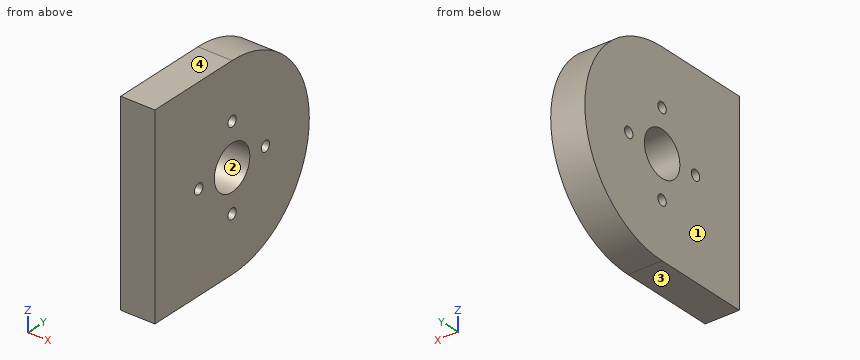
from build123d import *

# Parameters (mm, degrees)
SKETCH1_W               = 50
SKETCH1_H               = 150
BOSS_EXTRUDE1_DEPTH     = 55
CUT_EXTRUDE1_DEPTH      = 168.406690428
CUT_EXTRUDE1_DEPTH_BACK = 45
SKETCH2_R               = 10.25
SKETCH7_R               = 1
SKETCH7_R_2             = 4.25
CUT_EXTRUDE3_DEPTH      = 10
SKETCH8_W               = 55
SKETCH8_H               = 55
SKETCH8_R               = 10.25
BOSS_EXTRUDE2_DEPTH     = 50
SKETCH10_W              = 8
SKETCH10_H              = 10.25
SKETCH10_W_2            = 17
SKETCH10_H_2            = 1
SKETCH10_W_3            = 34
SKETCH10_H_3            = 20
SKETCH10_H_4            = 5
CUT_EXTRUDE4_DEPTH      = 214.717102732
SKETCH11_W              = 34
SKETCH11_H              = 13.25
BOSS_EXTRUDE4_DEPTH     = 25
SKETCH13_W              = 55
SKETCH13_H              = 10
CUT_EXTRUDE5_DEPTH      = 8
SKETCH14_R              = 5.030159043
CUT_EXTRUDE6_DEPTH      = 8
SKETCH15_W              = 34
SKETCH15_H              = 0.25
BOSS_EXTRUDE5_DEPTH     = 13.25
CUT_EXTRUDE7_DEPTH      = 181.416185527
BOSS_EXTRUDE6_START     = 1.5
SKETCH19_R              = 10.25
SKETCH19_R_2            = 1
SKETCH19_R_3            = 4.25
BOSS_EXTRUDE6_DEPTH     = 1.5
CUT_EXTRUDE8_DEPTH      = 184.89467094
SKETCH21_R              = 5.030159043
SKETCH21_R_2            = 4.5
BOSS_EXTRUDE7_DEPTH     = 8
SKETCH24_W              = 4
SKETCH24_H              = 30
CUT_EXTRUDE10_DEPTH     = 181.416185527
SKETCH25_W              = 55
SKETCH25_H              = 86.25
CUT_EXTRUDE11_DEPTH     = 4
BOSS_EXTRUDE8_START     = 4
SKETCH26_R              = 1
SKETCH26_R_2            = 4.25
BOSS_EXTRUDE8_DEPTH     = 4
SKETCH27_W              = 4
SKETCH27_H              = 123.25
CUT_EXTRUDE12_DEPTH     = 181.416185527
CUT_EXTRUDE13_DEPTH     = 180.905530765
SKETCH29_W              = 42
SKETCH29_H              = 9
CUT_EXTRUDE15_DEPTH     = 174.776436838
SKETCH30_R              = 4.5
SKETCH30_R_2            = 1.45
BOSS_EXTRUDE9_DEPTH     = 4
SKETCH31_W              = 37
SKETCH31_H              = 55
CUT_EXTRUDE16_DEPTH     = 182.05247858
SKETCH32_W              = 73.968301754
SKETCH32_H              = 92.223299302
CUT_EXTRUDE17_DEPTH     = 182.05247858


with BuildPart() as part:
    # Sketch1 → Boss-Extrude1 (new body)
    with BuildSketch(Plane.XY):
        with Locations((0, -75)):
            Rectangle(SKETCH1_W, SKETCH1_H)
    extrude(amount=-BOSS_EXTRUDE1_DEPTH)

    # Sketch2 → Cut-Extrude1 (cut, two sides: drawn at the far end of the back side and taken through both)
    with BuildSketch(Plane(origin=(25, 0, 0), x_dir=(0, 0, -1), z_dir=(1, 0, 0)).offset(-CUT_EXTRUDE1_DEPTH_BACK)):
        with Locations(Location((27.5, -25, 0), (0, 0, 270))):
            Circle(SKETCH2_R)
    extrude(amount=CUT_EXTRUDE1_DEPTH + CUT_EXTRUDE1_DEPTH_BACK, mode=Mode.SUBTRACT)

    # Sketch7 → Cut-Extrude3 (cut)
    with BuildSketch(Plane(origin=(-20, 0, 0), x_dir=(0, 0, -1), z_dir=(1, 0, 0))):
        with Locations(Location((27.5, -17, 0), (0, 0, 90))):
            Circle(SKETCH7_R)
        with Locations(Location((35.5, -25, 0), (0, 0, 90))):
            Circle(SKETCH7_R)
        with Locations(Location((27.5, -33, 0), (0, 0, 90))):
            Circle(SKETCH7_R)
        with Locations(Location((19.5, -25, 0), (0, 0, 90))):
            Circle(SKETCH7_R)
        with Locations(Location((27.5, -25, 0), (0, 0, 90))):
            Circle(SKETCH7_R_2)
    extrude(amount=-CUT_EXTRUDE3_DEPTH, mode=Mode.SUBTRACT)

    # Sketch8 → Boss-Extrude2 (add)
    with BuildSketch(Plane(origin=(25, 0, 0), x_dir=(0, 0, -1), z_dir=(1, 0, 0))):
        with Locations((27.5, -177.5)):
            Rectangle(SKETCH8_W, SKETCH8_H)
        with Locations(Location((27.5, -180, 0), (0, 0, 90))):
            Circle(SKETCH8_R, mode=Mode.SUBTRACT)
    extrude(amount=-BOSS_EXTRUDE2_DEPTH)

    # Sketch10 → Cut-Extrude4 (cut, through all)
    with BuildSketch(Plane.XY):
        Polygon((-17, -205), (17, -205), (17, -191.25), (0, -191.25), (-17, -191.25), align=None)
        Polygon((-25, -205), (-17, -205), (-17, -191.25), (-17, -190.25), (-25, -190.25), align=None)
        Polygon((17, -191.25), (17, -205), (25, -205), (25, -190.25), (17, -190.25), align=None)
        with Locations((-21, -185.125)):
            Rectangle(SKETCH10_W, SKETCH10_H)
        with Locations((-21, -174.875)):
            Rectangle(SKETCH10_W, SKETCH10_H)
        with Locations((21, -174.875)):
            Rectangle(SKETCH10_W, SKETCH10_H)
        with Locations((21, -185.125)):
            Rectangle(SKETCH10_W, SKETCH10_H)
        with Locations((-8.5, -185.125)):
            Rectangle(SKETCH10_W_2, SKETCH10_H)
        with Locations((8.5, -185.125)):
            Rectangle(SKETCH10_W_2, SKETCH10_H)
        Polygon((0, -180), (17, -180), (17, -169.75), (-17, -169.75), (-17, -180), align=None)
        with Locations((-8.5, -190.75)):
            Rectangle(SKETCH10_W_2, SKETCH10_H_2)
        with Locations((8.5, -190.75)):
            Rectangle(SKETCH10_W_2, SKETCH10_H_2)
        with Locations((0, -154.75)):
            Rectangle(SKETCH10_W_3, SKETCH10_H_3)
        with Locations((0, -167.25)):
            Rectangle(SKETCH10_W_3, SKETCH10_H_4)
    extrude(amount=-CUT_EXTRUDE4_DEPTH, mode=Mode.SUBTRACT)

    # Sketch11 → Boss-Extrude4 (add)
    with BuildSketch(Plane.XZ.offset(144.75)):
        with Locations((0, -6.625)):
            Rectangle(SKETCH11_W, SKETCH11_H)
        with Locations((0, -48.375)):
            Rectangle(SKETCH11_W, SKETCH11_H)
    extrude(amount=BOSS_EXTRUDE4_DEPTH)

    # Sketch13 → Cut-Extrude5 (cut)
    with BuildSketch(Plane(origin=(25, 0, 0), x_dir=(0, 0, -1), z_dir=(1, 0, 0))):
        with Locations((27.5, -164.75)):
            Rectangle(SKETCH13_W, SKETCH13_H)
    cut_extrude5 = extrude(amount=-CUT_EXTRUDE5_DEPTH, mode=Mode.SUBTRACT)

    # Mirror2: Cut-Extrude5 across plane
    add(cut_extrude5.mirror(Plane(origin=(0, 0, 0), x_dir=(0, 0, 1), z_dir=(1, 0, 0))), mode=Mode.SUBTRACT)

    # Sketch14 → Cut-Extrude6 (cut)
    with BuildSketch(Plane(origin=(25, 0, 0), x_dir=(0, 0, -1), z_dir=(1, 0, 0))):
        with Locations(Location((16.5, -148, 0), (0, 0, 90))):
            Circle(SKETCH14_R)
        with Locations(Location((38.5, -148, 0), (0, 0, 90))):
            Circle(SKETCH14_R)
    cut_extrude6 = extrude(amount=-CUT_EXTRUDE6_DEPTH, mode=Mode.SUBTRACT)

    # Mirror3: Cut-Extrude6 across plane
    add(cut_extrude6.mirror(Plane(origin=(0, 0, 0), x_dir=(0, 0, 1), z_dir=(1, 0, 0))), mode=Mode.SUBTRACT)

    # Sketch15 → Boss-Extrude5 (add)
    with BuildSketch(Plane.XY):
        with Locations((0, -169.875)):
            Rectangle(SKETCH15_W, SKETCH15_H)
    boss_extrude5 = extrude(amount=-BOSS_EXTRUDE5_DEPTH)

    # Mirror4: Boss-Extrude5 across plane
    add(boss_extrude5.mirror(Plane.XY.offset(-27.5)))

    # Sketch16 → Cut-Extrude7 (cut, through all)
    with BuildSketch(Plane.XY):
        Polygon((-18.5, 0), (-18.5, -14.75), (-18.5, -35.25), (-18.5, -43.5), (25, -43.5), (25, 0), align=None)
    extrude(amount=-CUT_EXTRUDE7_DEPTH, mode=Mode.SUBTRACT)

    # Sketch19 → Boss-Extrude6 (add)
    with BuildSketch(Plane(origin=(-20, 0, 0), x_dir=(0, 0, -1), z_dir=(1, 0, 0)).offset(BOSS_EXTRUDE6_START)):
        with Locations((27.5, -25)):
            Circle(SKETCH19_R)
        with Locations(Location((27.5, -17, 0), (0, 0, 90))):
            Circle(SKETCH19_R_2, mode=Mode.SUBTRACT)
        with Locations(Location((27.5, -33, 0), (0, 0, 90))):
            Circle(SKETCH19_R_2, mode=Mode.SUBTRACT)
        with Locations(Location((19.5, -25, 0), (0, 0, 90))):
            Circle(SKETCH19_R_2, mode=Mode.SUBTRACT)
        with Locations(Location((35.5, -25, 0), (0, 0, 90))):
            Circle(SKETCH19_R_2, mode=Mode.SUBTRACT)
        with Locations(Location((27.5, -25, 0), (0, 0, 90))):
            Circle(SKETCH19_R_3, mode=Mode.SUBTRACT)
    extrude(amount=-BOSS_EXTRUDE6_DEPTH)

    # Sketch20 → Cut-Extrude8 (cut, through all)
    with BuildSketch(Plane(origin=(-18.5, 0, 0), x_dir=(0, 0, -1), z_dir=(1, 0, 0))):
        with BuildLine():
            Line((0, 0), (0, -43.5))
            Line((0, -43.5), (9, -43.5))
            Line((9, -43.5), (9, -25))
            ThreePointArc((9, -25), (27.5, -6.5), (46, -25))
            Line((46, -25), (46, -43.5))
            Line((46, -43.5), (55, -43.5))
            Line((55, -43.5), (55, 0))
            Line((55, 0), (0, 0))
        make_face()
    extrude(amount=-CUT_EXTRUDE8_DEPTH, mode=Mode.SUBTRACT)

    # Sketch21 → Boss-Extrude7 (add)
    # profile 1 of 2: a face of its own
    with BuildSketch(Plane(origin=(25, 0, 0), x_dir=(0, 0, -1), z_dir=(1, 0, 0))):
        with Locations(Location((16.5, -148, 0), (0, 0, 229.751587581))):
            Circle(SKETCH21_R)
        with Locations(Location((16.5, -148, 0), (0, 0, 90))):
            Circle(SKETCH21_R_2, mode=Mode.SUBTRACT)
    # profile 2 of 2: a face of its own
    with BuildSketch(Plane(origin=(25, 0, 0), x_dir=(0, 0, -1), z_dir=(1, 0, 0))):
        with Locations(Location((38.5, -148, 0), (0, 0, 310.248412419))):
            Circle(SKETCH21_R)
        with Locations(Location((38.5, -148, 0), (0, 0, 90))):
            Circle(SKETCH21_R_2, mode=Mode.SUBTRACT)
    boss_extrude7 = extrude(amount=-BOSS_EXTRUDE7_DEPTH)

    # Mirror5: Boss-Extrude7 across plane
    add(boss_extrude7.mirror(Plane(origin=(0, 0, 0), x_dir=(0, 0, 1), z_dir=(1, 0, 0))))

    # Sketch24 → Cut-Extrude10 (cut, through all)
    with BuildSketch(Plane.XY):
        with Locations((-23, -144.75)):
            Rectangle(SKETCH24_W, SKETCH24_H)
        with Locations((23, -144.75)):
            Rectangle(SKETCH24_W, SKETCH24_H)
    extrude(amount=-CUT_EXTRUDE10_DEPTH, mode=Mode.SUBTRACT)

    # Sketch25 → Cut-Extrude11 (cut)
    with BuildSketch(Plane(origin=(25, 0, 0), x_dir=(0, 0, -1), z_dir=(1, 0, 0))):
        with Locations((27.5, -86.625)):
            Rectangle(SKETCH25_W, SKETCH25_H)
    extrude(amount=-CUT_EXTRUDE11_DEPTH, mode=Mode.SUBTRACT)

    # Sketch26 → Boss-Extrude8 (add)
    with BuildSketch(Plane(origin=(-18.5, 0, 0), x_dir=(0, 0, -1), z_dir=(1, 0, 0)).offset(BOSS_EXTRUDE8_START)):
        with BuildLine():
            Line((46, -43.5), (46, -25))
            ThreePointArc((46, -25), (27.5, -6.5), (9, -25))
            Line((9, -25), (9, -43.5))
            Line((9, -43.5), (46, -43.5))
        make_face()
        with Locations(Location((35.5, -25, 0), (0, 0, 90))):
            Circle(SKETCH26_R, mode=Mode.SUBTRACT)
        with Locations(Location((27.5, -25, 0), (0, 0, 90))):
            Circle(SKETCH26_R_2, mode=Mode.SUBTRACT)
        with Locations(Location((19.5, -25, 0), (0, 0, 90))):
            Circle(SKETCH26_R, mode=Mode.SUBTRACT)
        with Locations(Location((27.5, -33, 0), (0, 0, 90))):
            Circle(SKETCH26_R, mode=Mode.SUBTRACT)
        with Locations(Location((27.5, -17, 0), (0, 0, 90))):
            Circle(SKETCH26_R, mode=Mode.SUBTRACT)
    extrude(amount=-BOSS_EXTRUDE8_DEPTH)

    # Sketch27 → Cut-Extrude12 (cut, through all)
    with BuildSketch(Plane.XY):
        with Locations((-23, -68.125)):
            Rectangle(SKETCH27_W, SKETCH27_H)
    extrude(amount=-CUT_EXTRUDE12_DEPTH, mode=Mode.SUBTRACT)

    # Sketch28 → Cut-Extrude13 (cut, through all)
    with BuildSketch(Plane.XY):
        with BuildLine():
            Line((21, -43.5), (-14.5, -43.5))
            ThreePointArc((-14.5, -43.5), (10.602290732, -53.897709268), (21, -79))
            Line((21, -79), (21, -43.5))
        make_face()
    extrude(amount=-CUT_EXTRUDE13_DEPTH, mode=Mode.SUBTRACT)

    # Sketch29 → Cut-Extrude15 (cut, through all)
    with BuildSketch(Plane.XZ.offset(170)):
        with Locations((0, -50.5)):
            Rectangle(SKETCH29_W, SKETCH29_H)
        with Locations((0, -4.5)):
            Rectangle(SKETCH29_W, SKETCH29_H)
    extrude(amount=-CUT_EXTRUDE15_DEPTH, mode=Mode.SUBTRACT)

    # Sketch30 → Boss-Extrude9 (add)
    # profile 1 of 2: a face of its own
    with BuildSketch(Plane(origin=(21, 0, 0), x_dir=(0, 0, -1), z_dir=(1, 0, 0))):
        with Locations(Location((16.5, -148, 0), (0, 0, 223.761742693))):
            Circle(SKETCH30_R)
        with Locations((16.5, -148)):
            Circle(SKETCH30_R_2, mode=Mode.SUBTRACT)
    # profile 2 of 2: a face of its own
    with BuildSketch(Plane(origin=(21, 0, 0), x_dir=(0, 0, -1), z_dir=(1, 0, 0))):
        with Locations(Location((38.5, -148, 0), (0, 0, 316.238257307))):
            Circle(SKETCH30_R)
        with Locations((38.5, -148)):
            Circle(SKETCH30_R_2, mode=Mode.SUBTRACT)
    boss_extrude9 = extrude(amount=-BOSS_EXTRUDE9_DEPTH)

    # Mirror6: Boss-Extrude9 across plane
    add(boss_extrude9.mirror(Plane(origin=(0, 0, 0), x_dir=(0, 0, 1), z_dir=(1, 0, 0))))

    # Sketch31 → Cut-Extrude16 (cut, through all)
    with BuildSketch(Plane.ZY.offset(21)):
        with Locations((-27.5, -71)):
            Rectangle(SKETCH31_W, SKETCH31_H)
    extrude(amount=-CUT_EXTRUDE16_DEPTH, mode=Mode.SUBTRACT)


with BuildPart() as cut_extrude16_piece_1:
    # of the separate pieces the step leaves, piece 1, a body of its own (cut_extrude16_pieces)
    add(part.part.solids().sort_by_distance((17, -170, -13.25))[0])

    # Sketch32 → Cut-Extrude17 (cut, through all)
    with BuildSketch(Plane.ZY.offset(21)):
        with Locations((-28.833527464, -129.267729309)):
            Rectangle(SKETCH32_W, SKETCH32_H)
    extrude(amount=-CUT_EXTRUDE17_DEPTH, mode=Mode.SUBTRACT)


with BuildPart() as cut_extrude16_piece_2:
    # of the separate pieces the step leaves, piece 2, a body of its own (cut_extrude16_pieces)
    add(part.part.solids().sort_by_distance((-21, -43.5, -9))[0])


solid = cut_extrude16_piece_2.part
The listing builds one solid part. Answer for the finished solid, in the listing's coordinates (mm). Face numbers are marked on the shaded views. Coordinates: 2 decimals unless noted, no trailing zeros. Order: outer loops, then holes, each group sorted by start corner. A loop starts at its lowest first (then second) coordinate and runs counter-clockwise, first axis right, second up.
Q1. A cutting plane is placed at D-D, the plane z = -19.5. Write down the section's boundary in (x, y).
Q2. Consider line 1 (Z direction, x = -15.75, y = -25); line 2 (Z direction, x = -19.5, y = -33); line 3 (Y direction, x = -14.75, z = -20). Determine where each line is inside the solid, lowest interval first.
Q3. A cutting plane is placed at C-C, the plane y = -17. Write down the section's boundary in (x, z).
Q4. A cutting plane is placed at B-B, the plane x = -15.25. Write down the section's boundary in (y, z).
Q5. Given P1, Ø3, axis at x = -18.5, z = -23, coming from the +Y side; P2, Ø2, axis at x = -20, z = -13, coming from the +Y side, each flat-ended and moving along its own axis, determine where each tip first touches the part or whether it passes through.
Q6. For a pull along Z with two mould halves and no side action, classify the marked faces 1, 2, 3 and 4 as pulls with the +Z half, pulls with the -Z half, needs draft (parallel to the pull), parting line crosses it, or undercut.
Q7. A cutting plane is placed at A-A, the plane z = -27.5. Write down the section's boundary in (x, y).
Answers follow:
1. outline: (-21, -43.5) - (-14.5, -43.5) - (-14.5, -26) - (-21, -26) - close; (-21, -24) - (-14.5, -24) - (-14.5, -8.32) - (-21, -8.32) - close
2. line 1: z = -46 to -36.5, -34.5 to -31.75, -23.25 to -20.5, -18.5 to -9
2. line 2: z = -46 to -28.5, -26.5 to -9
2. line 3: y = -43.5 to -25.87, -24.13 to -8.09
3. outline: (-21, -44.18) - (-14.5, -44.18) - (-14.5, -28.5) - (-21, -28.5) - close; (-21, -26.5) - (-14.5, -26.5) - (-14.5, -10.82) - (-21, -10.82) - close
4. outline: (-43.5, -46) - (-25, -46) arc R18.5 ccw to (-25, -9) - (-43.5, -9) - close; hole circle Ø2 at (-33, -27.5); hole circle Ø8.5 at (-25, -27.5); hole circle Ø2 at (-25, -35.5); hole circle Ø2 at (-25, -19.5); hole circle Ø2 at (-17, -27.5)
5. P1: stops at y = -6.74
5. P2: stops at y = -12.35
6. face 1: needs draft
6. face 2: undercut
6. face 3: pulls with the -Z half
6. face 4: pulls with the +Z half
7. outline: (-21, -43.5) - (-14.5, -43.5) - (-14.5, -34) - (-21, -34) - close; (-21, -32) - (-14.5, -32) - (-14.5, -29.25) - (-21, -29.25) - close; (-21, -20.75) - (-14.5, -20.75) - (-14.5, -18) - (-21, -18) - close; (-21, -16) - (-14.5, -16) - (-14.5, -6.5) - (-21, -6.5) - close
